```python
from build123d import *

# Parameters (mm, degrees)
SKETCH1_R           = 30.0863
BOSS_EXTRUDE1_DEPTH = 6.35
SKETCH2_R           = 36.5125
BOSS_EXTRUDE2_DEPTH = 25.4
SKETCH3_R           = 19.05
BOSS_EXTRUDE3_DEPTH = 38.1
DRAFT1_ANGLE        = 15
SKETCH4_R           = 19.05
BOSS_EXTRUDE4_DEPTH = 25.4
CHAMFER1_SIZE       = 2.54
FILLET1_R           = 6.35
CHAMFER2_SIZE       = 1.5875


with BuildPart() as part:
    # Sketch1 → Boss-Extrude1 (new body)
    with BuildSketch(Plane.XY):
        Circle(SKETCH1_R)
    extrude(amount=-BOSS_EXTRUDE1_DEPTH)

    # Sketch2 → Boss-Extrude2 (add)
    with BuildSketch(Plane.XY):
        Circle(SKETCH2_R)
    extrude(amount=BOSS_EXTRUDE2_DEPTH)

    # Sketch3 → Boss-Extrude3 (add)
    with BuildSketch(Plane.XY.offset(25.4)):
        Circle(SKETCH3_R)
    extrude(amount=BOSS_EXTRUDE3_DEPTH)

    # Draft1
    draft1_faces = [part.faces().sort_by_distance(p)[0] for p in [
        (-19.05, 0, 44.45),
    ]]
    draft(draft1_faces, Plane.XY.offset(63.5), DRAFT1_ANGLE)

    # Sketch4 → Boss-Extrude4 (add)
    with BuildSketch(Plane.XY.offset(63.5)):
        Circle(SKETCH4_R)
    extrude(amount=BOSS_EXTRUDE4_DEPTH)

    # Chamfer1
    chamfer1_edges = [part.edges().sort_by_distance(p)[0] for p in [
        (-19.05, 0, 88.9),
    ]]
    chamfer(chamfer1_edges, length=CHAMFER1_SIZE)

    # Fillet1
    fillet1_edges = [part.edges().sort_by_distance(p)[0] for p in [
        (-19.05, 0, 63.5),
        (-29.258864232, 0, 25.4),
    ]]
    fillet(fillet1_edges, radius=FILLET1_R)

    # Chamfer2
    chamfer2_edges = [part.edges().sort_by_distance(p)[0] for p in [
        (-36.5125, 0, 25.4),
    ]]
    chamfer(chamfer2_edges, length=CHAMFER2_SIZE)


solid = part.part
```
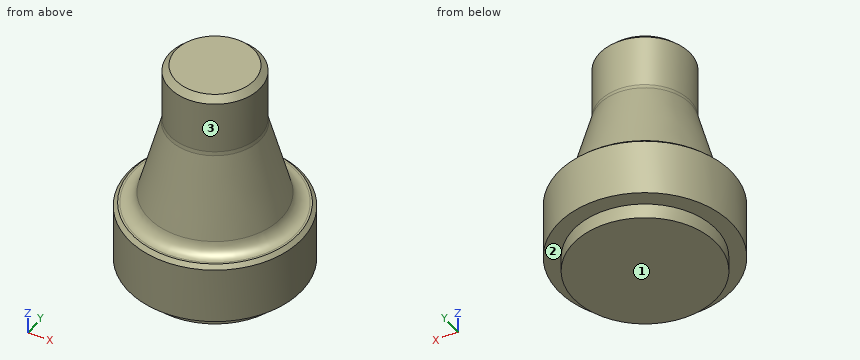
The model under review builds one solid part; all positions refer to its coordinate system, in mm. Face numbers are marked on the shaded views. A direction names the side the tool comes from. Coordinates: 2 decimals unless noted, no trailing zeros. Write each loop counter-clockwise with the first axis right and the second up, starting at its lowest first coordinate (ties: lowest second). Pieces come first, ordered by that corner, then holes. Notation, with made-up numbers: (42.5, 45) - (95.5, 45) arc R20 ccw to (95.5, 79) - close; hole circle Ø11 at (17, -7.75). An arc over 180 degrees is marked (long way). Write item = value, one per line.
(1) For P1, Ø6, axis at x = 7.5, z = 32, coming from the +Y side; P2, Ø6, axis at y = -3, z = 10.5, coming from the -X side; P3, Ø3, axis at y = 14.5, z = 56, coming from the +X side; P4, Ø12, axis at y = 15, z = 10, coming from the +X side, all flat-tipped, find the tip position at first contact; note any pin that passes through.
Result sheet:
P1 = 27.59
P2 = -36.51
P3 = 16.67
P4 = 35.39
(2) For line 1 (Z direction, x = 9, y = 33); line 2 (Y direction, x = -10, z = 68); line 3 (X direction, y = 8.5, z = 3), list the stretches that pass through material, from the lowest coordinate up. Write a range as [from, to].
Result sheet:
line_1 = [0, 25.4]
line_2 = [-16.21, 16.21]
line_3 = [-35.51, 35.51]
(3) Consider section B-B, the plane z = 2.5. Give the boundary of the cut face in (x, y) (1 decimal), then the cut area to 3 significant figures.
Result sheet:
outline = circle Ø73 at (0, 0)
area = 4,190 mm^2
(4) Machinability: for the marked faces 1, 2 and 3, which of the approach directions +Z, -Z, +X, -X, +Y, -Y give a long, thin tool a straight path to every point of the face, cutting with its end or side? Answer none if there is none.
Result sheet:
face_1 = -Z, +X, -X, +Y, -Y
face_2 = -Z
face_3 = +Z
(5) Consider section A-A, the plane z = 72.5. Give the boundary of the cut face in (x, y), then the cut area to 3 significant figures.
Result sheet:
outline = circle Ø38.1 at (0, 0)
area = 1,140 mm^2
